Answer from the drawing. Dimensions are ordinates in mm from the lowest x, y and z of the part. Give positions to 0.01 mm unless a question says otherwise; leave off trailing zeros. Write each loop counter-clockwise with the first axis right and the second up, starting at its lowest first coordinate (ties: lowest second). Pieces come first, ordered by that corner, then holes. Notation, with made-up numbers: (-22.75, 15) -> (34.25, 15) arc R8 cw to (34.25, 23) -> close; hole circle Ø11 at (50, 53.25). An arc over 180 degrees is marked (long way). Put each result on its own line as item: value. Start each with the question number.
1) Flat-ended cylindrical pins translate along their axes: pin 1 Ø1.5 at (x, z) = (1, 2) entering from -Y; pin 2 Ø1.5 at (y, z) = (14, 1) entering from -X; pin 3 Ø1.5 at (y, z) = (1.5, 1.5) entering from +X. Find the tip coordinate at first contact, or state that the pin passes through.
2) Find the intervals of material crossed by line 1 along Y through (x, z) = (23, 1.95); line 2 along X through (y, z) = (31.5, 0.8); line 3 along Y through (x, z) = (20.5, 2.3), in increasing order. Write a range as from..to.
3) A cutting plane is placed at C-C (x = 23). Write down the section's boundary in (y, z).
4) A cutting plane is placed at A-A (y = 13). Write down the section's boundary in (x, z), then the cut area to 3 significant figures.
5) A cutting plane is placed at B-B (x = 37). Write down the section's boundary in (y, z).
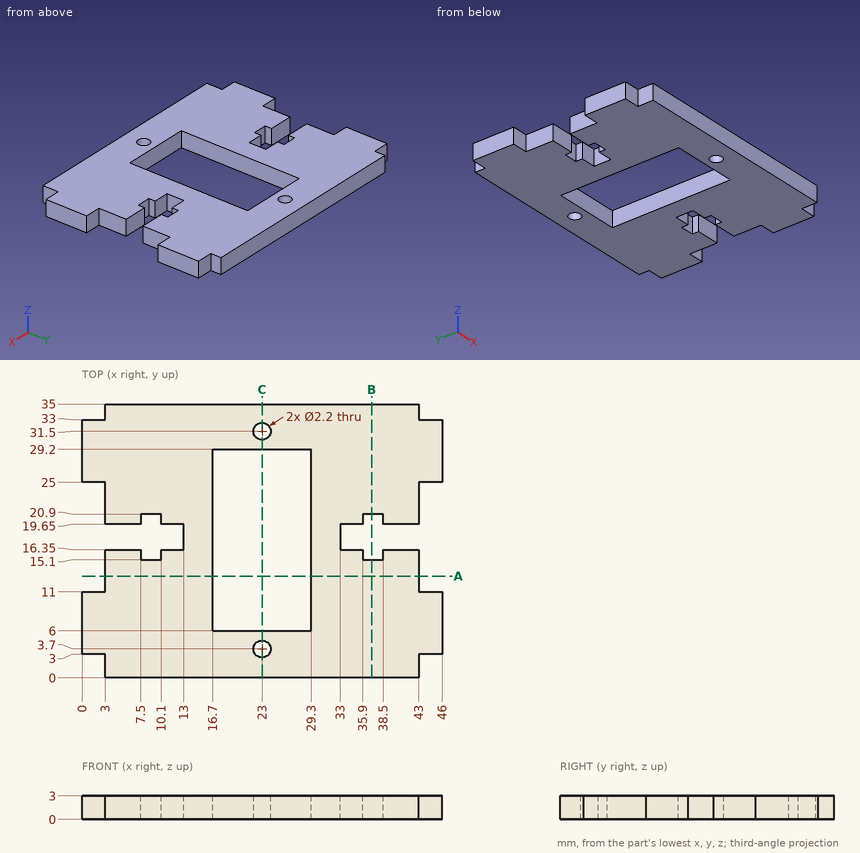
Reply:
1. pin 1: stops at y = 3
1. pin 2: stops at x = 3
1. pin 3: stops at x = 43
2. line 1: y = 0..2.6, 4.8..6, 29.2..30.4, 32.6..35
2. line 2: x = 0..21.9, 24.1..46
2. line 3: y = 0..6, 29.2..35
3. outline: (0, 0) -> (2.6, 0) -> (2.6, 3) -> (0, 3) -> close; (4.8, 0) -> (6, 0) -> (6, 3) -> (4.8, 3) -> close; (29.2, 0) -> (30.4, 0) -> (30.4, 3) -> (29.2, 3) -> close; (32.6, 0) -> (35, 0) -> (35, 3) -> (32.6, 3) -> close
4. outline: (3, 0) -> (16.7, 0) -> (16.7, 3) -> (3, 3) -> close; (29.3, 0) -> (43, 0) -> (43, 3) -> (29.3, 3) -> close
4. area: 82.2 mm2
5. outline: (0, 0) -> (15.1, 0) -> (15.1, 3) -> (0, 3) -> close; (20.9, 0) -> (35, 0) -> (35, 3) -> (20.9, 3) -> close
